Check sheet for the drawn part. Datum: minimum x, y, z corner. Units: mm. Coordinates: 2 decimals unless noted, no trailing zeros. Write each loop counter-clockwise with the first axis right and the second up, starting at its lowest first coordinate (ties: lowest second). Pieces come first, ordered by that corner, then holes. Notation, with made-up numbers: (-18.5, 39) -> (4.5, 39) arc R24 cw to (4.5, 74) -> close; hole circle Ø3 at (26, 61.5). An arc over 180 degrees is marked (long way). Answer in a Markdown table with one row per item. Add a question column.
1. Cross-section at C-C on y = 1.25. Record the cut outline in (x, z).
2. Depth check by flat-ended pin: P1, Ø3, axis at x = 87.5, z = 87.5, coming from the -Y side. Enter the tip coordinate at first touch or a pass-through.
3. Cross-section at A-A on z = 22.86. Record the cut outline in (x, y) (3 decimals).
4. Scan lines: L1, parallel to X at y = 1.5, z = 76.2; L2, parallel to Z at x = 104, y = 2.5; L3, parallel to X at y = 2, z = 71.5. Record each from-to range of solid material in increasing order. Write a range as from..to.
5. Cross-section at B-B on z = 71. Record the cut outline in (x, y) (3 decimals), and give its area (3 significant figures).
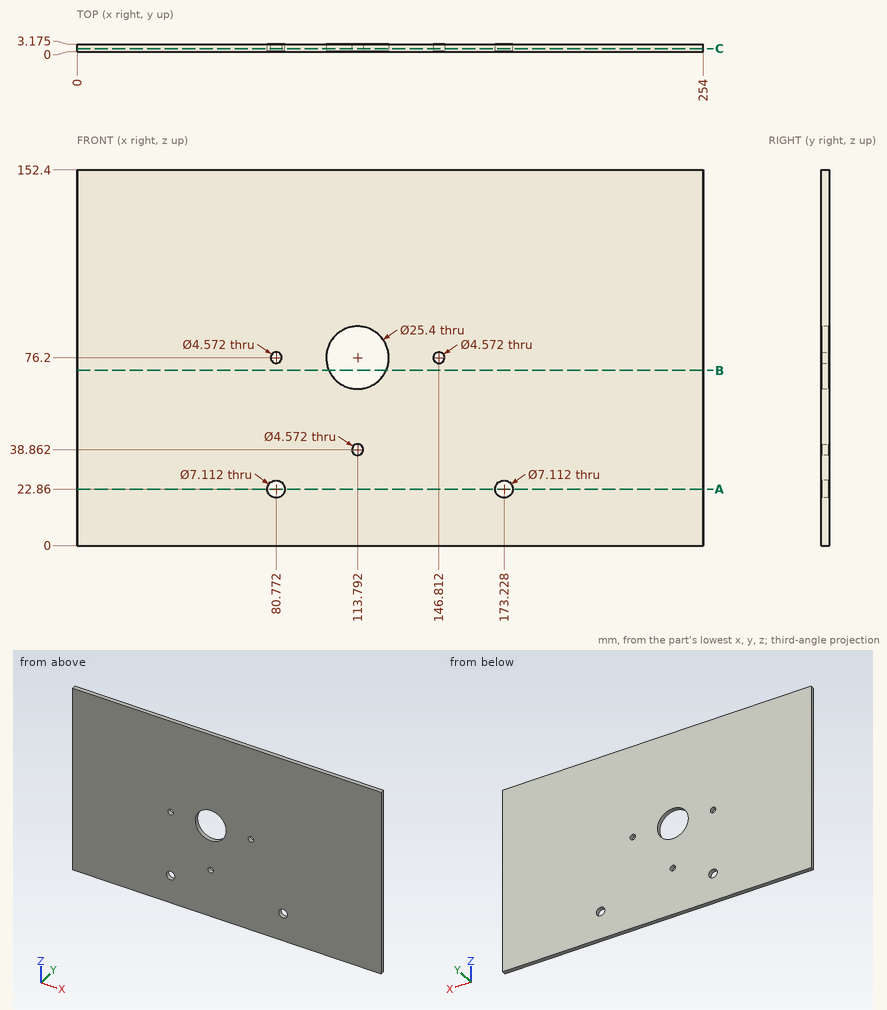
Results found:
| question | item | result |
|---|---|---|
| 1 | outline | (0, 0) -> (254, 0) -> (254, 152.4) -> (0, 152.4) -> close; hole circle Ø7.11 at (80.77, 22.86); hole circle Ø4.57 at (80.77, 76.2); hole circle Ø25.4 at (113.79, 76.2); hole circle Ø4.57 at (113.79, 38.86); hole circle Ø4.57 at (146.81, 76.2); hole circle Ø7.11 at (173.23, 22.86) |
| 2 | P1 | stops at y = 0 |
| 3 | outline | (0, 0) -> (77.216, 0) -> (77.216, 3.175) -> (0, 3.175) -> close; (84.328, 0) -> (169.672, 0) -> (169.672, 3.175) -> (84.328, 3.175) -> close; (176.784, 0) -> (254, 0) -> (254, 3.175) -> (176.784, 3.175) -> close |
| 4 | L1 | x = 0..78.49, 83.06..101.09, 126.49..144.53, 149.1..254 |
| 4 | L2 | z = 0..68.11, 84.29..152.4 |
| 4 | L3 | x = 0..101.99, 125.59..254 |
| 5 | outline | (0, 0) -> (102.205, 0) -> (102.205, 3.175) -> (0, 3.175) -> close; (125.379, 0) -> (254, 0) -> (254, 3.175) -> (125.379, 3.175) -> close |
| 5 | area | 733 mm^2 |
